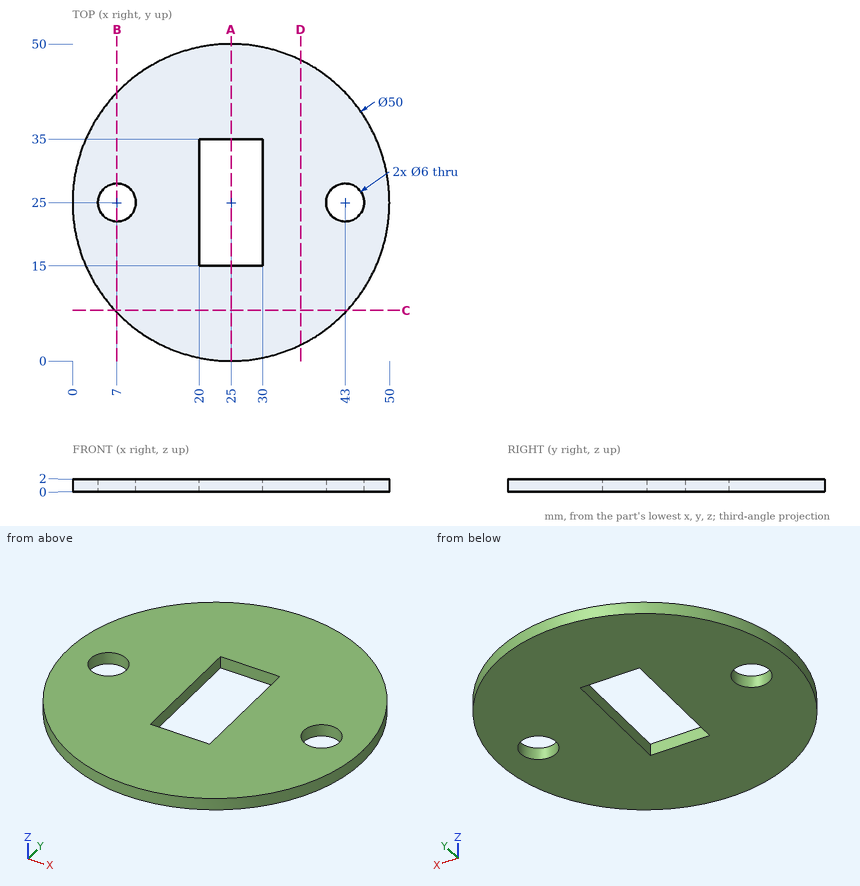
Could you check a few things on this drawing? It's one solid part, dimensions in mm from its lowest x, y, z. Give positions to 0.01 mm unless a question says otherwise; leave off trailing zeros. Write each loop counter-clockwise with the first axis right and the second up, starting at its lowest first coordinate (ties: lowest second). Pieces come first, ordered by that corner, then holes.
(1) Will these pins go through, and if not, where does the flat tip stop? pin 1 (1 mm diameter, centred on x = 26, z = 1, fed in from +Y) (3 decimals); pin 2 (1 mm diameter, centred on y = 23.5, z = 1, fed in from +X); pin 3 (1 mm diameter, centred on y = 22.5, z = 1, fed in from -X); pin 4 (3.5 mm diameter, centred on x = 43, y = 25, fed in from -Z).
Output values:
pin 1: stops at y = 49.995
pin 2: stops at x = 49.98
pin 3: stops at x = 0.08
pin 4: passes through
(2) If I drill on L1, parallel to Y at x = 25.5, z = 0.75 (3 decimals); L2, parallel to X at y = 23, z = 0.45; L3, parallel to Y at x = 7, z = 0.55, over which ranges is the centre line in solid material (lowest first)?
Output values:
L1: y = 0.005 to 15, 35 to 49.995
L2: x = 0.08 to 4.76, 9.24 to 20, 30 to 40.76, 45.24 to 49.92
L3: y = 7.65 to 22, 28 to 42.35
(3) Imagine slicing it at C-C, the plane y = 8. Write out the boundary of the cut face in (x, z).
Output values:
outline: (6.67, 0) - (43.33, 0) - (43.33, 2) - (6.67, 2) - close
(4) Imagine slicing it at D-D, the plane x = 36. Write out the boundary of the cut face in (y, z).
Output values:
outline: (2.55, 0) - (47.45, 0) - (47.45, 2) - (2.55, 2) - close
(5) Imagine slicing it at A-A, the plane x = 25. Write out the boundary of the cut face in (y, z), and give its area (3 significant figures).
Output values:
outline: (0, 0) - (15, 0) - (15, 2) - (0, 2) - close; (35, 0) - (50, 0) - (50, 2) - (35, 2) - close
area: 60.0 mm2
(6) Imagine slicing it at B-B, the plane x = 7. Write out the boundary of the cut face in (y, z).
Output values:
outline: (7.65, 0) - (22, 0) - (22, 2) - (7.65, 2) - close; (28, 0) - (42.35, 0) - (42.35, 2) - (28, 2) - close
